Design review of the part built by this model. Coordinates are the model's own, in mm. A direction names the side the tool comes from. Give positions to 0.01 mm unless a question says otherwise; leave off trailing zeros. Loops run counter-clockwise (first coordinate to the right, second up) from the corner with the lowest first, then second, coordinate; pieces in that order, holes last.
from build123d import *

# Parameters (mm, degrees)
SKETCH1_W           = 304.8
SKETCH1_H           = 304.8
BOSS_EXTRUDE1_DEPTH = 19.05
SKETCH2_W           = 254
SKETCH2_H           = 254
CUT_EXTRUDE1_DEPTH  = 18.796
SKETCH3_W           = 279.4
SKETCH3_H           = 279.4
CUT_EXTRUDE2_DEPTH  = 11.684


with BuildPart() as part:
    # Sketch1 → Boss-Extrude1 (new body)
    with BuildSketch(Plane.XY):
        Rectangle(SKETCH1_W, SKETCH1_H)
    extrude(amount=BOSS_EXTRUDE1_DEPTH)

    # Sketch2 → Cut-Extrude1 (cut)
    with BuildSketch(Plane(origin=(0, 0, 0), x_dir=(-1, 0, 0), z_dir=(0, 0, -1))):
        Rectangle(SKETCH2_W, SKETCH2_H)
    extrude(amount=-CUT_EXTRUDE1_DEPTH, mode=Mode.SUBTRACT)

    # Sketch3 → Cut-Extrude2 (cut)
    with BuildSketch(Plane(origin=(0, 0, 18.796), x_dir=(-1, 0, 0), z_dir=(0, 0, -1))):
        Rectangle(SKETCH3_W, SKETCH3_H)
    extrude(amount=CUT_EXTRUDE2_DEPTH, mode=Mode.SUBTRACT)


solid = part.part
Q1. Wall thickness on line 1 (X direction, y = 40.5, z = 8.25); line 2 (Y direction, x = -7, z = 1.75): over which ranges is each line inside the solid? List them lowest first.
Results:
line 1: x = -152.4 to -139.7, 139.7 to 152.4
line 2: y = -152.4 to -127, 127 to 152.4
Q2. Draft analysis for pull direction X (two halves, no side actions). For faces 4 (the face through (127, -2, 4)), 5 (the face through (-152.4, -2, 9)), 6 (the face through (-2, 2, 19.05)), state which applies: pulls with the +X half, pulls with the -X half, needs draft (parallel to the pull), parting line crosses it, or undercut.
Results:
face 4: undercut
face 5: pulls with the -X half
face 6: needs draft
Q3. Take a section at B-B (x = 115.5). Give the boundary of the cut face in (y, z), plus the area to 3 significant figures.
Results:
outline: (-152.4, 0) - (-127, 0) - (-127, 7.11) - (-139.7, 7.11) - (-139.7, 18.8) - (139.7, 18.8) - (139.7, 7.11) - (127, 7.11) - (127, 0) - (152.4, 0) - (152.4, 19.05) - (-152.4, 19.05) - close
area: 735 mm2
Q4. Tool access review of faces 1 (the face through (2, 127, 4)), 2 (the face through (-139.7, -2, 13)), 3 (the face through (152.4, -2, 9)): name each direction out of +Z, -Z, +X, -X, +Y, -Y from which nothing blocks a thin tool from reaching the whole face with its end or side.
Results:
face 1: -Z
face 2: none
face 3: +Z, -Z, +X, +Y, -Y
Q5. Take a section at A-A (z = 3.75). Give the boundary of the cut face in (x, y).
Results:
outline: (-152.4, -152.4) - (152.4, -152.4) - (152.4, 152.4) - (-152.4, 152.4) - close; hole (-127, -127) - (127, -127) - (127, 127) - (-127, 127) - close
Q6. Insertion check: pin 1 (1 mm diameter, centred on x = -1.5, y = 88.5, fed in from -Z). The pin has a flat end and moves straight along its axis. Give the tip position at first contact, or say it passes through.
Results:
pin 1: stops at z = 18.8
